Can you work these out from the model? Positions are in its coordinate system, mm. A direction names the side the tool comes from. Give positions to 0.01 mm unless a question says otherwise; leave off trailing zeros. Loops run counter-clockwise (first coordinate to the right, second up) from the corner with the lowest first, then second, coordinate; pieces in that order, holes last. Notation, with made-up numbers: (-13, 37) -> (7, 37) arc R25 ccw to (7, 57) -> close; hole circle Ø7 at (17.25, 48.5). An arc over 180 degrees is marked (long way). Use CSV: the item, a comma, the result in double quotes.
from build123d import *

# Parameters (mm, degrees)
F1_DEPTH      = 327.025
F2_R          = 4.7625
F3_DEPTH      = 50.801
F4_R          = 3.175
F5_DEPTH      = 50.801
F5_DEPTH_BACK = 697


# Not quite as in the source:
# - an extrude ends at something that could not be found from the text; its depth is read off the source's solid


with BuildPart() as f1:
    # F0 (on Right) → F1 (new body, symmetric)
    with BuildSketch(Plane.YZ):
        Polygon((0, 44.45), (0, 0), (6.35, 0), (6.35, 50.8), (-44.45, 50.8), (-44.45, 44.45), align=None)
    extrude(amount=F1_DEPTH, both=True)

    # F2 (on face) → F3 (cut, through all)
    with BuildSketch(Plane.XY.offset(50.8)):
        with Locations((-285.75, -31.75)):
            Circle(F2_R)
        with Locations((-95.25, -31.75)):
            Circle(F2_R)
        with Locations((95.25, -31.75)):
            Circle(F2_R)
        with Locations((285.75, -31.75)):
            Circle(F2_R)
    extrude(amount=-F3_DEPTH, mode=Mode.SUBTRACT)

    # F4 (on face) → F5 (cut, two sides)
    with BuildSketch(Plane(origin=(0, 6.35, 0), x_dir=(-1, 0, 0), z_dir=(0, 1, 0))) as f5_sk:
        with Locations((209.55, 15.24)):
            Circle(F4_R)
        with Locations((171.45, 15.24)):
            Circle(F4_R)
        with Locations((19.05, 15.24)):
            Circle(F4_R)
        with Locations((-19.05, 15.24)):
            Circle(F4_R)
        with Locations((-171.45, 15.24)):
            Circle(F4_R)
        with Locations((-209.55, 15.24)):
            Circle(F4_R)
    extrude(amount=-F5_DEPTH, mode=Mode.SUBTRACT)
    extrude(f5_sk.sketch, amount=F5_DEPTH_BACK, mode=Mode.SUBTRACT)


solid = f1.part
(1) If I drill on L1, parallel to Z at x = 209, y = 4; L2, parallel to Y at x = 286, z = 14; L3, parallel to Z at x = -259.5, y = -13, over which ranges is the centre line in solid material (lowest first)? Write a range as from..to.
Answer sheet:
L1,"z = 0..12.11, 18.37..50.8"
L2,"y = 0..6.35"
L3,"z = 44.45..50.8"
(2) If we section it at A-A, the plane x = 190.5: Write out the boundary of the cut face in (y, z).
Answer sheet:
outline,"(-44.45, 44.45) -> (0, 44.45) -> (0, 0) -> (6.35, 0) -> (6.35, 50.8) -> (-44.45, 50.8) -> close"
(3) Which directions (+Z, -Z, +X, -X, +Y, -Y) give clear straight access to the entire face, cutting with the end or side of a thin tool? Please do faces 1 (the face through (5, -23, 44.45)), 2 (the face through (5, 6.35, 25)).
Answer sheet:
face 1,"-Z, +X, -X, -Y"
face 2,"+Z, -Z, +X, -X, +Y"
(4) Will these pins go through, and if not, where does the flat tip stop? pin 1 Ø6 at (x, z) = (113.5, 15.5) entering from -Y; pin 2 Ø5.5 at (x, z) = (-19.05, 15.24) entering from +Y; pin 3 Ø10 at (x, y) = (-85, -21.5) entering from -Z.
Answer sheet:
pin 1,"stops at y = 0"
pin 2,"passes through"
pin 3,"stops at z = 44.45"
(5) If we section it at B-B, the plane y = -8: Write out the boundary of the cut face in (x, z) (3 decimals), then the cut area to 3 significant figures.
Answer sheet:
outline,"(-327.025, 44.45) -> (327.025, 44.45) -> (327.025, 50.8) -> (-327.025, 50.8) -> close"
area,"4,150 mm2"
